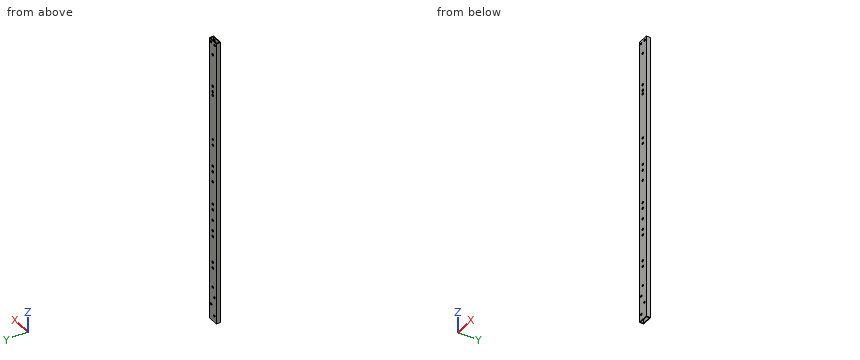
from build123d import *

# Parameters (mm, degrees)
SKETCH_1_W          = 15
SKETCH_1_H          = 6
SKETCH_1_W_2        = 13
SKETCH_1_H_2        = 4
EXTRUDE_1_DEPTH     = 400
SKETCH_2_R          = 1.5
CUT_EXTRUDE_1_DEPTH = 10
SKETCH_3_R          = 1.6
SKETCH_3_R_2        = 1.55
CUT_EXTRUDE_2_DEPTH = 10
SKETCH_4_R          = 1.55
SKETCH_4_R_2        = 1.5
CUT_EXTRUDE_3_DEPTH = 401.115295884


with BuildPart() as part:
    # 草图1 → 凸台-拉伸1 (new body)
    with BuildSketch(Plane.XY):
        Rectangle(SKETCH_1_W, SKETCH_1_H)
        Rectangle(SKETCH_1_W_2, SKETCH_1_H_2, mode=Mode.SUBTRACT)
    extrude(amount=EXTRUDE_1_DEPTH)

    # 草图2 → 切除-拉伸1 (cut)
    with BuildSketch(Plane.XZ.offset(3)):
        with Locations(Location((-3.5, 35, 0), (0, 0, 270))):
            Circle(SKETCH_2_R)
        with Locations(Location((-3.5, 9, 0), (0, 0, 270))):
            Circle(SKETCH_2_R)
        with Locations(Location((3.5, 22, 0), (0, 0, 270))):
            Circle(SKETCH_2_R)
        with Locations(Location((0, 48, 0), (0, 0, 270))):
            Circle(SKETCH_2_R)
    extrude(amount=-CUT_EXTRUDE_1_DEPTH, mode=Mode.SUBTRACT)

    # 草图3 → 切除-拉伸2 (cut)
    with BuildSketch(Plane(origin=(0, 3, 0), x_dir=(1, 0, 0), z_dir=(0, 1, 0))):
        with Locations(Location((0, -322, 0), (0, 0, 270))):
            Circle(SKETCH_3_R)
        with Locations(Location((0, -327, 0), (0, 0, 270))):
            Circle(SKETCH_3_R)
        with Locations(Location((0, -335, 0), (0, 0, 270))):
            Circle(SKETCH_3_R)
        with Locations(Location((0, -380, 0), (0, 0, 270))):
            Circle(SKETCH_3_R)
        with Locations(Location((0, -213, 0), (0, 0, 270))):
            Circle(SKETCH_3_R)
        with Locations(Location((0, -221, 0), (0, 0, 270))):
            Circle(SKETCH_3_R)
        with Locations(Location((0, -198.5, 0), (0, 0, 270))):
            Circle(SKETCH_3_R_2)
        with Locations(Location((0, -158.5, 0), (0, 0, 270))):
            Circle(SKETCH_3_R)
        with Locations(Location((0, -143.5, 0), (0, 0, 270))):
            Circle(SKETCH_3_R)
        with Locations(Location((0, -128.5, 0), (0, 0, 270))):
            Circle(SKETCH_3_R)
        with Locations(Location((0, -120.5, 0), (0, 0, 270))):
            Circle(SKETCH_3_R)
        with Locations(Location((0, -75.5, 0), (0, 0, 270))):
            Circle(SKETCH_3_R)
        with Locations(Location((0, -83.5, 0), (0, 0, 270))):
            Circle(SKETCH_3_R)
    extrude(amount=-CUT_EXTRUDE_2_DEPTH, mode=Mode.SUBTRACT)

    # 草图4 → 切除-拉伸3 (cut, through all)
    with BuildSketch(Plane(origin=(0, 3, 0), x_dir=(1, 0, 0), z_dir=(0, 1, 0))):
        with Locations(Location((0, -251.1, 0), (0, 0, 270))):
            Circle(SKETCH_4_R)
        with Locations(Location((0, -259.1, 0), (0, 0, 270))):
            Circle(SKETCH_4_R)
        with Locations(Location((0, -166.6, 0), (0, 0, 270))):
            Circle(SKETCH_4_R)
        with Locations(Location((-4, -396, 0), (0, 0, 270))):
            Circle(SKETCH_4_R_2)
        with Locations(Location((4, -396, 0), (0, 0, 270))):
            Circle(SKETCH_4_R_2)
    extrude(amount=-CUT_EXTRUDE_3_DEPTH, mode=Mode.SUBTRACT)


solid = part.part
The model under review builds one solid part; all positions refer to its coordinate system, in mm. Round coordinates to 2 decimals unless told otherwise and drop trailing zeros. Write each loop counter-clockwise with the first axis right and the second up, starting at its lowest first coordinate (ties: lowest second). Pieces come first, ordered by that corner, then holes. Notation, with made-up numbers: M -15,-20.75 L 17,-20.75 A33 ccw 17,8.25 Z; hole C -4,-11.5 d3. An arc over 180 degrees is marked long. Answer as CSV lines item,"result". Start each with the question number.
Q1. Consider section A-A, the plane y = -0.95. Give the boundary of the cut face in (x, z), then the cut area to 3 significant figures.
Q2. Consider section B-B, the plane z = 304. Give the boundary of the cut face in (x, y).
Q3. Clearance check with flat-ended pins moving along their axes: P1, Ø4, axis at x = 0, z = 75.5, coming from the +Y side; P2, Ø1, axis at x = 2.5, y = -1, coming from the -Z side. State where each tip first meets the part, or that it passes through.
Q4. Wall thickness on line 1 along X through (y, z) = (-2.55, 396); line 2 along X through (y, z) = (-1.25, 319); line 3 along X through (y, z) = (-2.4, 83.5): over which ranges is each line inside the solid? List them lowest first.
Result set:
1,outline,"M -7.5,0 L -6.5,0 L -6.5,400 L -7.5,400 Z; M 6.5,0 L 7.5,0 L 7.5,400 L 6.5,400 Z"
1,area,"800 mm²"
2,outline,"M -7.5,-3 L 7.5,-3 L 7.5,3 L -7.5,3 Z; hole M -6.5,-2 L 6.5,-2 L 6.5,2 L -6.5,2 Z"
3,P1,"stops at y = 3"
3,P2,"passes through"
4,line 1,"x = -7.5 to -5.5, -2.5 to 2.5, 5.5 to 7.5"
4,line 2,"x = -7.5 to -6.5, 6.5 to 7.5"
4,line 3,"x = -7.5 to -1.6, 1.6 to 7.5"
